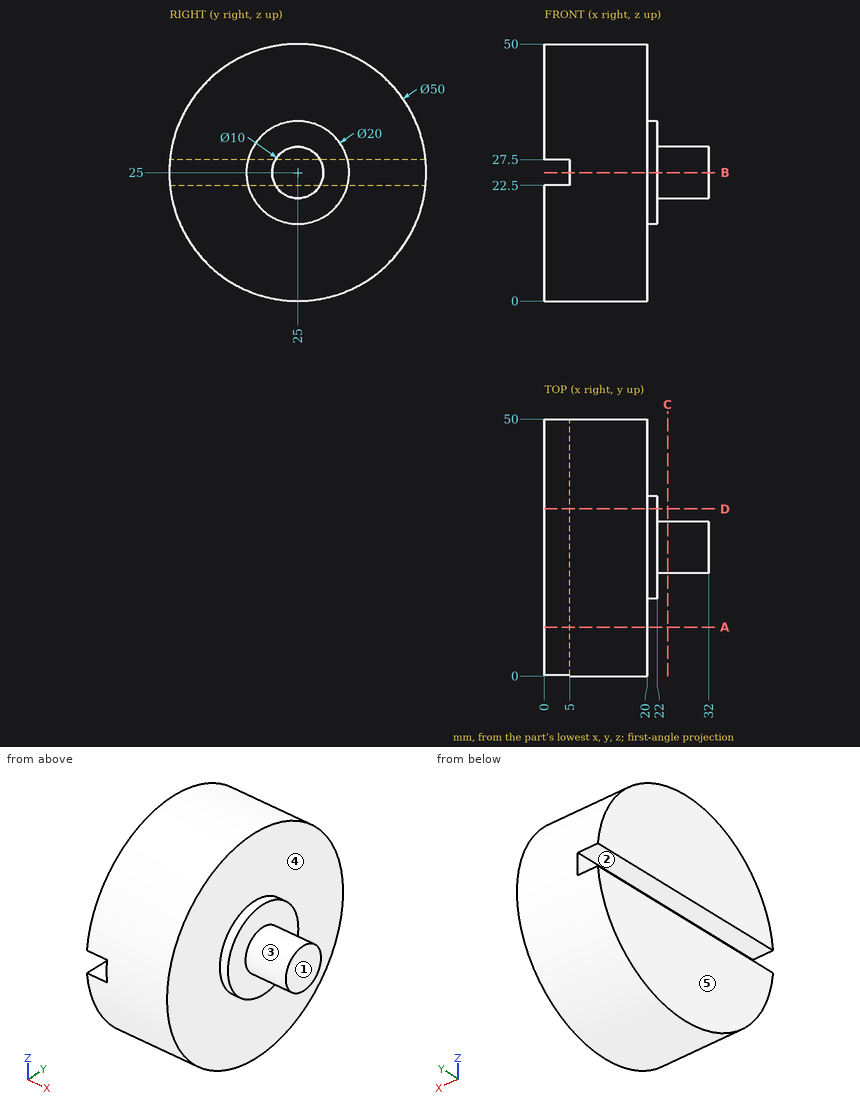
Can you work these out from the drawing? Everything is in mm from the part's minimum corner. A direction names the side the tool comes from. Give positions to 0.01 mm unless a question says otherwise; leave off trailing zeros. Order: outer loops, then holes, each group sorted by start corner. A loop starts at its lowest first (then second) coordinate and runs counter-clockwise, first axis right, second up. Notation, with made-up numbers: M -17,12.25 L 20,12.25 A26 cw 20,30.25 Z; hole C -25.5,31 d5. An arc over 180 degrees is marked long. Use a Markdown table: item, result. Add a question column.
1. On a 3-axis mill with a long thin cutter (end or side, diameter ignored), from which of +Z, -Z, +X, -X, +Y, -Y can I reach the whole of each face in a straight line? I mean the marked faces 4 and 5. Say none if no direction works.
2. Suppose I cut it at C-C (x = 24). List the corners of the cut face in (y, z) for me, and give its area (3 significant figures).
3. If we mould it in two halves opening along Z, with no side actions, what happens to the marked faces 1, 2 and 3? For each: +Z half, -Z half, draft (parallel to the pull), parting line (faces both ways), or undercut.
4. For pin 1 Ø10 at (x, z) = (17, 8.5) entering from +Y; pin 2 Ø8 at (x, z) = (13.5, 9) entering from -Y; pin 3 Ø8 at (x, y) = (23, 14.5) entering from +Z, each with a flat end and sliding along its axis, tell me the tip position at first contact or that it passes through.
5. Suppose I cut it at A-A (y = 9.5). List the corners of the cut face in (x, z) for me.
6. Suppose I cut it at D-D (y = 32.5). List the corners of the cut face in (x, z) for me.
7. I need wall thicknesses on probe 1 along X at (y, z) = (25.5, 39); probe 2 along X at (y, z) = (18, 21); probe 3 along Z at (x, y) = (2, 23). Which ranges of each line are inside material? Lowest first, please. Write a range as from..to.
8. Suppose I cut it at B-B (z = 25). List the corners of the cut face in (x, y) for me.
Results list:
| question | item | result |
|---|---|---|
| 1 | face 4 | +X |
| 1 | face 5 | +Z, -Z, -X, +Y, -Y |
| 2 | outline | C 25,25 d10 |
| 2 | area | 78.5 mm² |
| 3 | face 1 | draft |
| 3 | face 2 | undercut |
| 3 | face 3 | parting line |
| 4 | pin 1 | stops at y = 47.2 |
| 4 | pin 2 | stops at y = 3.07 |
| 4 | pin 3 | stops at z = 48.73 |
| 5 | outline | M 0,5.38 L 20,5.38 L 20,44.62 L 0,44.62 L 0,27.5 L 5,27.5 L 5,22.5 L 0,22.5 Z |
| 6 | outline | M 0,1.15 L 20,1.15 L 20,18.39 L 22,18.39 L 22,31.61 L 20,31.61 L 20,48.85 L 0,48.85 L 0,27.5 L 5,27.5 L 5,22.5 L 0,22.5 Z |
| 7 | probe 1 | x = 0..20 |
| 7 | probe 2 | x = 0..22 |
| 7 | probe 3 | z = 0.08..22.5, 27.5..49.92 |
| 8 | outline | M 5,0 L 20,0 L 20,15 L 22,15 L 22,20 L 32,20 L 32,30 L 22,30 L 22,35 L 20,35 L 20,50 L 5,50 Z |
